Geometry: final body of the model. Coordinates: model frame, mm. Face numbers are marked on the shaded views. A direction names the side the tool comes from. Round coordinates to 2 decimals unless told otherwise and drop trailing zeros. Loops run counter-clockwise (first coordinate to the right, second up) from the corner with the lowest first, then second, coordinate; pieces in that order, holes last. Notation, with made-up numbers: (76.25, 19) - (109.25, 19) arc R27 cw to (109.25, 54) - close; hole circle Ø10 at (89, 80). An arc over 180 degrees is marked (long way). Answer as CSV lines item,"result".
from build123d import *

# Parameters (mm, degrees)
F0_R     = 14.414674
F1_DEPTH = 50.8
F2_W     = 12.7
F2_H     = 12.7
F3_DEPTH = 12.7
F5_DEPTH = 38.1


with BuildPart() as f1:
    # F0 (on Right) → F1 (new body)
    with BuildSketch(Plane.YZ):
        with Locations((-56.139331, 5.552941)):
            Circle(F0_R)
    extrude(amount=-F1_DEPTH)

    # F2 (on face) → F3 (cut)
    with BuildSketch(Plane.YZ):
        with Locations((-56.067919, 5.498222)):
            Rectangle(F2_W, F2_H)
    extrude(amount=-F3_DEPTH, mode=Mode.SUBTRACT)

    # F4 (on face) → F5 (cut, through all)
    with BuildSketch(Plane(origin=(-50.8, 0, 0), x_dir=(0, -1, 0), z_dir=(-1, 0, 0))):
        Polygon((62.867289, -2.07704), (66.111067, 7.564533), (59.383109, 15.194513), (49.411373, 13.182921), (46.167595, 3.541348), (52.895554, -4.088632), align=None)
    extrude(amount=-F5_DEPTH, mode=Mode.SUBTRACT)


solid = f1.part
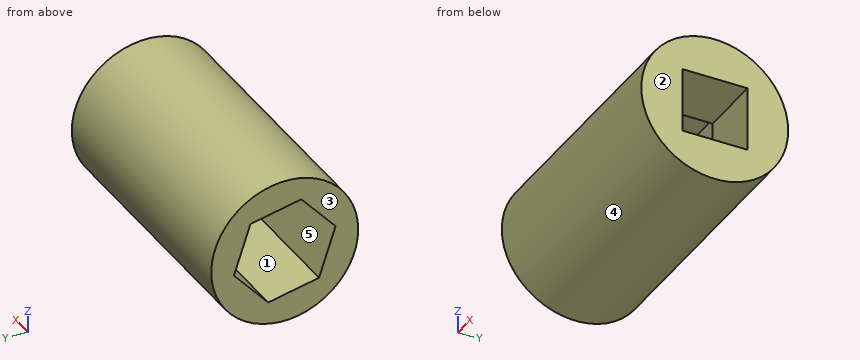
(1) Section B-B (z = 8.5). Output: boundary loops of the cut face in (x, y), and give its area (3 significant figures).
Findings below:
outline,"(-50.8, -70.25) - (0, -70.25) - (0, -62.42) - (-12.7, -62.42) - (-12.7, -65.29) - (-50.8, -65.29) - close; (-50.8, -47.84) - (-12.7, -47.84) - (-12.7, -49.72) - (0, -49.72) - (0, -42.03) - (-50.8, -42.03) - close"
area,"607 mm2"
(2) Section C-C (y = -50.75). Output: boundary loops of the cut face in (x, z), and give its area (3 significant figures).
Findings below:
outline,"(-50.8, -7.82) - (0, -7.82) - (0, -0.85) - (-12.7, -0.85) - (-12.7, -1.66) - (-50.8, -1.66) - close; (-50.8, 13.45) - (-12.7, 13.45) - (-12.7, 11.85) - (0, 11.85) - (0, 18.92) - (-50.8, 18.92) - close"
area,"621 mm2"
(3) Pin query (flat end, axial travel): P1, Ø4, axis at x = -9.5, y = -54.5, coming from the +Z side; P2, Ø1, axis at x = -12, z = 11, coming from the +Y side; P3, Ø2, axis at x = -6, y = -54, coming from the +Z side; P4, Ø1.5, axis at x = -35, z = 15.5, coming from the -Y side. Return the tip coordinate at first contact, or that it passes through.
Findings below:
P1,"z = 19.97"
P2,"y = -42.6"
P3,"z = 19.92"
P4,"y = -67.24"
(4) Material intervals for line 1 along Z through (x, y) = (-47, -54); line 2 along Z through (x, y) = (-17, -50); line 3 along X through (y, z) = (-57.75, -2.25), sorted ascending.
Findings below:
line 1,"-8.7 to -3.87, 14.11 to 19.81"
line 2,"-7.49 to -0.8, 13.3 to 18.59"
line 3,"-12.7 to 0"
(5) Section A-A (x = -2.5). Output: boundary loops of the cut face in (y, z).
Findings below:
outline,"circle Ø28.83 at (-56.14, 5.55); hole (-62.42, -0.85) - (-49.72, -0.85) - (-49.72, 11.85) - (-62.42, 11.85) - close"
(6) Section D-D (z = 14). Output: boundary loops of the cut face in (x, y), and give its area (3 significant figures).
Findings below:
outline,"(-50.8, -67.82) - (0, -67.82) - (0, -44.46) - (-50.8, -44.46) - (-50.8, -53.46) - (-12.7, -53.46) - (-12.7, -60.44) - (-50.8, -60.44) - close"
area,"921 mm2"
(7) Access query for the marked faces 1 and 2. Directions: +Z, -Z, +X, -X, +Y, -Y. A direction counts if a zero-diameter tool reaches every point of the face in a straight line with its end or side. Return the directions, or none.
Findings below:
face 1,"-X"
face 2,"+Z, -Z, +X, +Y, -Y"
(8) Draft query along Y for the marked faces 3, 4 and 5. Return one class per face: pulls with the +Y half, pulls with the -Y half, needs draft (parallel to the pull), parting line crosses it, or undercut.
Findings below:
face 3,"needs draft"
face 4,"parting line crosses it"
face 5,"undercut"
